```python
from build123d import *

# Parameters (mm, degrees)
F0_W     = 115.471501
F0_H     = 32.801882
F1_DEPTH = 19.05
F2_W     = 115.249865
F2_H     = 14.627867
F3_DEPTH = 50.8
F4_W     = 12.7
F4_H     = 15.24
F5_DEPTH = 19.05


with BuildPart() as f1:
    # F0 (on Front) → F1 (new body)
    with BuildSketch(Plane.XZ):
        with Locations((0.110819, -13.962963)):
            Rectangle(F0_W, F0_H)
    extrude(amount=F1_DEPTH)

    # F2 (on Front) → F3 (join)
    with BuildSketch(Plane.XZ):
        with Locations((0.221636, -22.828339)):
            Rectangle(F2_W, F2_H)
    extrude(amount=F3_DEPTH)

    # F4 (on face) → F5 (cut)
    with BuildSketch(Plane(origin=(0, 0, 0), x_dir=(-1, 0, 0), z_dir=(0, 1, 0))):
        with Locations((44.924932, -5.182022)):
            Rectangle(F4_W, F4_H)
        with Locations((25.874932, -5.182022)):
            Rectangle(F4_W, F4_H)
        with Locations((6.824932, -5.182022)):
            Rectangle(F4_W, F4_H)
        with Locations((-12.225068, -5.182022)):
            Rectangle(F4_W, F4_H)
        with Locations((-31.275068, -5.182022)):
            Rectangle(F4_W, F4_H)
        with Locations((-50.325068, -5.182022)):
            Rectangle(F4_W, F4_H)
    extrude(amount=-F5_DEPTH, mode=Mode.SUBTRACT)


solid = f1.part
```
Design review of the part built by this model. Coordinates are the model's own, in mm. A direction names the side the tool comes from. Coordinates: 2 decimals unless noted, no trailing zeros. Order: outer loops, then holes, each group sorted by start corner. A loop starts at its lowest first (then second) coordinate and runs counter-clockwise, first axis right, second up.
1) Wall thickness on line 1 along Z through (x, y) = (-37, -36); line 2 along X through (y, z) = (-29.5, -22); line 3 along Y through (x, z) = (44.5, -13): over which ranges is each line inside the solid? List them lowest first.
2) Take a section at A-A, the plane z = -3. Give the boundary of the cut face in (x, y), and give its area (3 significant figures).
3) For faces 4 (the flat face through (-57.403, -35, -23)), 5 (the flat face through (-32.225, -9, -5)), 6 (the flat face through (-1, -35, -15.514)), 7 (the flat face through (-1, -9, -30.364)), 8 (the flat face through (-1, -50.8, -23)), list the 3-axis set-ups (+Z, -Z, +X, -X, +Y, -Y) from which the entire face can be reached by the end or side of a thin tool; tool diameter is ignored.
4) Mouldability with a two-part tool opening along X and no side actions: class faces 1 (the flat face through (-1, -35, -30.142)), 2 (the flat face through (-57.625, -9, -14)), 3 (the flat face through (31, -9, -12.802)) as +X half, -X half, draft (parallel to the pull), parting line (faces both ways), or undercut.
5) Clearance check with flat-ended pins moving along their axes: pin 1 (12 mm diameter, centred on x = -29, z = -8.5, fed in from -Y); pin 2 (10 mm diameter, centred on y = -44.5, z = -19.5, fed in from -X); pin 3 (8 mm diameter, centred on x = 42.5, z = -12, fed in from -Y); pin 4 (3 mm diameter, centred on x = 15.5, y = -23, fed in from -Z). State where each tip first meets the part, or that it passes through.
6) Take a section at D-D, the plane x = 22.5. Give the boundary of the cut face in (y, z).
7) Take a section at C-C, the plane y = -17. Give the boundary of the cut face in (x, z).
8) Take a section at B-B, the plane x = -28. Give the boundary of the cut face in (y, z).
Returned:
1. line 1: z = -30.14 to -15.51
1. line 2: x = -57.4 to 57.85
1. line 3: y = -19.05 to 0
2. outline: (-57.62, -19.05) - (-51.27, -19.05) - (-51.27, 0) - (-57.62, 0) - close; (-38.57, -19.05) - (-32.22, -19.05) - (-32.22, 0) - (-38.57, 0) - close; (-19.52, -19.05) - (-13.17, -19.05) - (-13.17, 0) - (-19.52, 0) - close; (-0.47, -19.05) - (5.88, -19.05) - (5.88, 0) - (-0.47, 0) - close; (18.58, -19.05) - (24.93, -19.05) - (24.93, 0) - (18.58, 0) - close; (37.63, -19.05) - (43.98, -19.05) - (43.98, 0) - (37.63, 0) - close; (56.68, -19.05) - (57.85, -19.05) - (57.85, 0) - (56.68, 0) - close
2. area: 748 mm2
3. face 4: +Z, -Z, -X, -Y
3. face 5: +Z, +Y, -Y
3. face 6: +Z, +X, -X, -Y
3. face 7: -Z, +X, -X, +Y, -Y
3. face 8: +Z, -Z, +X, -X, -Y
4. face 1: draft
4. face 2: -X half
4. face 3: undercut
5. pin 1: stops at y = -19.05
5. pin 2: stops at x = -57.4
5. pin 3: stops at y = -50.8
5. pin 4: stops at z = -30.14
6. outline: (-50.8, -30.14) - (-19.05, -30.14) - (-19.05, -30.36) - (0, -30.36) - (0, 2.44) - (-19.05, 2.44) - (-19.05, -15.51) - (-50.8, -15.51) - close
7. outline: (-57.62, -30.36) - (57.85, -30.36) - (57.85, 2.44) - (56.68, 2.44) - (56.68, -12.8) - (43.98, -12.8) - (43.98, 2.44) - (37.63, 2.44) - (37.63, -12.8) - (24.93, -12.8) - (24.93, 2.44) - (18.58, 2.44) - (18.58, -12.8) - (5.88, -12.8) - (5.88, 2.44) - (-0.47, 2.44) - (-0.47, -12.8) - (-13.17, -12.8) - (-13.17, 2.44) - (-19.52, 2.44) - (-19.52, -12.8) - (-32.22, -12.8) - (-32.22, 2.44) - (-38.57, 2.44) - (-38.57, -12.8) - (-51.27, -12.8) - (-51.27, 2.44) - (-57.62, 2.44) - close
8. outline: (-50.8, -30.14) - (-19.05, -30.14) - (-19.05, -30.36) - (0, -30.36) - (0, -12.8) - (-19.05, -12.8) - (-19.05, -15.51) - (-50.8, -15.51) - close
